from build123d import *

# Parameters (mm, degrees)
PAD_DEPTH    = 25.4
POCKET_DEPTH = 23.4
FILLET_R     = 1


with BuildPart() as corner:
    # Sketch → Pad (new body)
    with BuildSketch(Plane.XY):
        with BuildLine():
            Line((0, 0), (0, -25.4))
            ThreePointArc((0, -25.4), (15.435414, -20.171961), (24.516737, -6.64))
            Line((0, 0), (24.516737, -6.64))
        make_face()
    extrude(amount=PAD_DEPTH)

    # Sketch001 (on Face5 of Pad) → Pocket (cut)
    with BuildSketch(Plane.XY.offset(25.4)):
        with BuildLine():
            Line((2, -2.5), (2, -27.9))
            ThreePointArc((2, -27.9), (17.435414, -22.671961), (26.516737, -9.14))
            Line((2, -2.5), (26.516737, -9.14))
        make_face()
    extrude(amount=-POCKET_DEPTH, mode=Mode.SUBTRACT)

    # Fillet
    fillet_edges = [corner.edges().sort_by_distance(p)[0] for p in [
        (0, -25.4, 12.7),
        (0, -12.7, 25.4),
        (0, -12.7, 0),
        (0, 0, 12.7),
        (15.435414, -20.171961, 0),
        (12.258369, -3.32, 0),
        (12.258369, -3.32, 25.4),
        (24.516737, -6.64, 12.7),
    ]]
    fillet(fillet_edges, radius=FILLET_R)


with BuildPart() as part_mirroring:
    # Part__Mirroring: instance of Corner
    add(corner.part.mirror(Plane(origin=(0, 0, 0), x_dir=(1, 0, 0), z_dir=(0, 1, 0))))


solid = part_mirroring.part
Verification items for the finished model (mm, model axes). A direction names the side the tool comes from. Coordinates: 2 decimals unless noted, no trailing zeros. Write each loop counter-clockwise with the first axis right and the second up, starting at its lowest first coordinate (ties: lowest second). Pieces come first, ordered by that corner, then holes. Notation, with made-up numbers: (49.5, 55.5) - (58.5, 55.5) arc R27 ccw to (58.5, 94.5) - close; hole circle Ø9 at (23.25, 55.5). An arc over 180 degrees is marked (long way). Answer as a JSON object with one key per item and string values.
(1) Gauge pin test, flat ends, axial feed: pin 1 Ø3 at (x, z) = (18.5, 14.5) entering from +Y; pin 2 Ø2 at (x, z) = (5.5, 21.5) entering from +Y; pin 3 Ø3 at (x, z) = (9, 14) entering from -Y. Record the tip position at first contact, or that the pin passes through.
Report:
{"pin 1": "y = 7.38", "pin 2": "y = 3.72", "pin 3": "y = 2.03"}
(2) Tool access check on faces 5 (the cylindrical face through (0.285, 13.512, 25.099)), 6 (the flat face through (10, 14, 2)). Record the directions out of +Z, -Z, +X, -X, +Y, -Y that give a thin tool (end or side, any length) a straight path to the whole face; none if there is none.
Report:
{"face 5": "+Z, -X, +Y, -Y", "face 6": "+Z, +Y"}
(3) Cross-section at A-A on z = 12. Record the cut outline in (x, y), plus the area to 3 significant figures.
Report:
{"outline": "(0, 1.31) arc R1 ccw to (1.26, 0.34) - (23.53, 6.37) arc R1 ccw to (24.22, 7.64) arc R25.4 ccw to (23.95, 8.45) - (2, 2.5) - (2, 25.32) arc R25.4 ccw to (1.04, 25.38) arc R1 ccw to (0, 24.38) - close", "area": "92.9 mm^2"}
(4) Thickness scan on line 1 along Z through (x, y) = (11.5, 16.25); line 2 along Y through (x, z) = (6.75, 19.75). Record the ranges inside material, lowest first.
Report:
{"line 1": "0 to 2", "line 2": "1.83 to 3.79"}
(5) Mould release check, pull along X, two halves, no side actions. Record for faces 1 (the flat face through (12.82, 5.43, 13.86)), 2 (the flat face through (2, 14, 14)), 3 (the cylindrical face through (15.4, 20.2, 1.4)), 4 (the cylindrical face through (0.285, 13.005, 0.301)): pulls with the +X half, pulls with the -X half, needs draft (parallel to the pull), parting line crosses it, or undercut.
Report:
{"face 1": "undercut", "face 2": "undercut", "face 3": "pulls with the +X half", "face 4": "pulls with the -X half"}
